Geometry check sheet. Reference: the model listing, model coordinates, mm. Face numbers are marked on the shaded views. A direction names the side the tool comes from. Round coordinates to 2 decimals unless told otherwise and drop trailing zeros. Order: outer loops, then holes, each group sorted by start corner. A loop starts at its lowest first (then second) coordinate and runs counter-clockwise, first axis right, second up.
(1) Sectioned sample at A-A (y = 60). Record the boundary of the cut face in (x, z), plus the area to 3 significant figures.
(2) Sectioned sample at B-B (x = -62). Record the boundary of the cut face in (y, z), plus the area to 3 significant figures.
(3) Release check for a two-part mould opening along Y. For the marked faces 1, 2, 3 and 4 record: +Y half, -Y half, draft (parallel to the pull), parting line (faces both ways), or undercut.
(4) Material ranges on line 1 along Z through (x, y) = (-64.5, 211), recorded low to high.
(5) Set-up check for the marked faces 5 and 6: record each of +Z, -Z, +X, -X, +Y, -Y from which the full face is reachable in a straight line by a thin tool's end or side.
(6) Sectioned sample at C-C (y = 176.5). Record the boundary of the cut face in (x, z), plus the area to 3 significant figures.
(7) Go/stop test with a flat-tipped pin: pin 1 (19 mm diameter, centred on x = 169.5, y = 216.5, fed in from +Z). Record where the tip stops, or that it passes through.
from build123d import *

# Parameters (mm, degrees)
SKETCH1_W           = 450
SKETCH1_H           = 290
BOSS_EXTRUDE1_DEPTH = 260
SKETCH2_R           = 31.915290565
SKETCH2_W           = 89.685507292
SKETCH2_H           = 39.972356382
SKETCH2_W_2         = 306.987697012
SKETCH2_H_2         = 209.632802358
CUT_EXTRUDE1_DEPTH  = 12


with BuildPart() as part:
    # Sketch1 → Boss-Extrude1 (new body)
    with BuildSketch(Plane(origin=(0, 0, 0), x_dir=(1, 0, 0), z_dir=(0, 1, 0))):
        Rectangle(SKETCH1_W, SKETCH1_H)
    extrude(amount=BOSS_EXTRUDE1_DEPTH)

    # Sketch2 → Cut-Extrude1 (cut)
    with BuildSketch(Plane.XY.offset(145)):
        with Locations((168.275900741, 203.066569732)):
            Circle(SKETCH2_R)
        with Locations((168.275900741, 126.418305405)):
            Circle(SKETCH2_R)
        with Locations((168.275900741, 47.697411123)):
            Rectangle(SKETCH2_W, SKETCH2_H)
        with Locations((-48.183132642, 129.533317372)):
            Rectangle(SKETCH2_W_2, SKETCH2_H_2)
    extrude(amount=-CUT_EXTRUDE1_DEPTH, mode=Mode.SUBTRACT)


solid = part.part
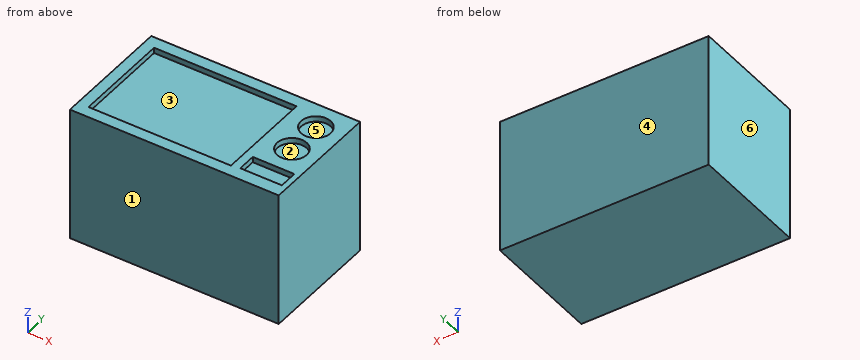
Answer below:
1. outline: (-225, -145) - (225, -145) - (225, 145) - (213.12, 145) - (213.12, 133) - (123.43, 133) - (123.43, 145) - (105.31, 145) - (105.31, 133) - (-201.68, 133) - (-201.68, 145) - (-225, 145) - close
1. area: 126,000 mm2
2. outline: (0, -145) - (260, -145) - (260, 145) - (234.35, 145) - (234.35, 133) - (24.72, 133) - (24.72, 145) - (0, 145) - close
2. area: 72,900 mm2
3. face 1: -Y half
3. face 2: undercut
3. face 3: undercut
3. face 4: +Y half
4. line 1: z = -145 to 133
5. face 5: +Z
5. face 6: +Z, -Z, -X, +Y, -Y
6. outline: (-225, -145) - (225, -145) - (225, 145) - (185.96, 145) - (185.96, 133) - (150.59, 133) - (150.59, 145) - (105.31, 145) - (105.31, 133) - (-201.68, 133) - (-201.68, 145) - (-225, 145) - close
6. area: 126,000 mm2
7. pin 1: stops at z = 133
